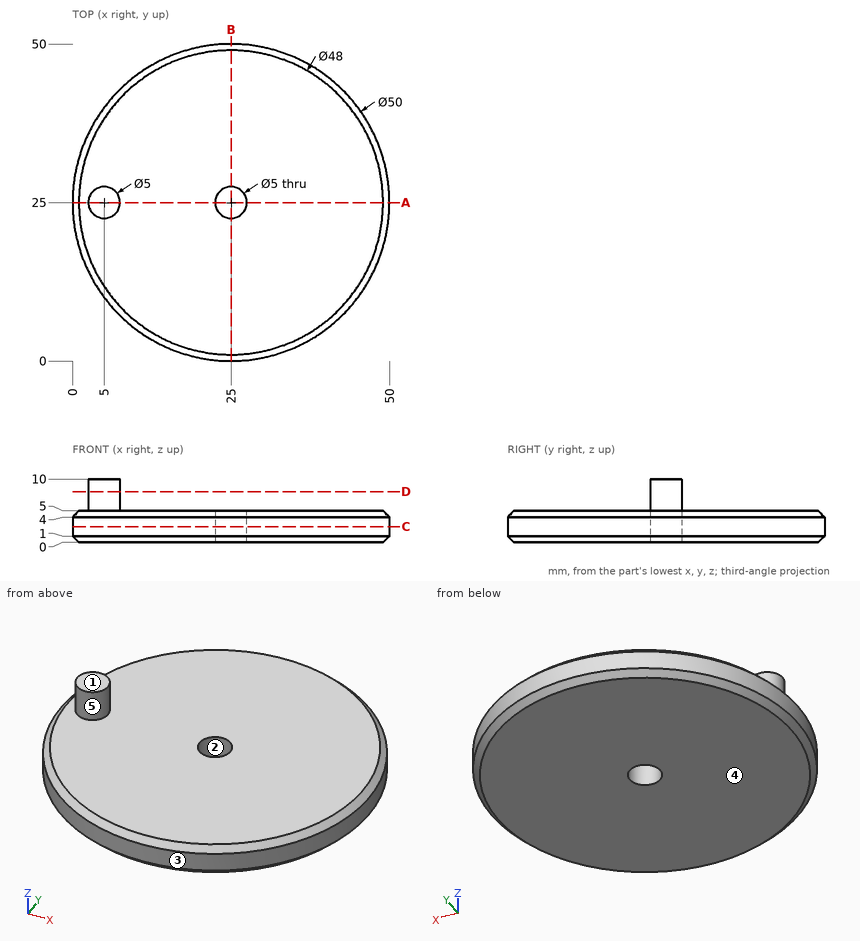
Here's the drawing with two shaded views (mm, measured from the low corner). I have some questions. A direction names the side the tool comes from. Give positions to 0.01 mm unless a question says otherwise; leave off trailing zeros. Loops run counter-clockwise (first coordinate to the right, second up) from the corner with the lowest first, then second, coordinate; pieces in that order, holes last. Notation, with made-up numbers: (63.25, 62) - (77.25, 62) arc R15 cw to (77.25, 78) - close; hole circle Ø11 at (84, 30.25). An arc over 180 degrees is marked (long way). One line per item, written item: value.
(1) If we section it at D-D, the plane z = 8: List the corners of the cut face in (x, y) for me, plus the area to 3 significant figures.
Verdict:
outline: circle Ø5 at (5, 25)
area: 19.6 mm^2
(2) If we mould it in two halves opening along Y, with no side actions, what happens to the marked faces 1, 2 and 3? For each: released by +Y, released by -Y, zero draft, split by the parting line, or undercut.
Verdict:
face 1: zero draft
face 2: undercut
face 3: split by the parting line
(3) I'm going to push flat-ended pins straight in: pin 1 (6 mm diameter, centred on x = 37.5, z = 5.5, fed in from -Y); pin 2 (2 mm diameter, centred on y = 27, z = 8, fed in from +X); pin 3 (3 mm diameter, centred on y = 34.5, z = 3.5, fed in from -X). Where does each tip first touch, or does it pass through?
Verdict:
pin 1: y = 2.04
pin 2: x = 7.29
pin 3: x = 1.31
(4) On a 3-axis mill with a long thin cutter (end or side, diameter ignored), from which of +Z, -Z, +X, -X, +Y, -Y can I reach the whole of each face in a straight line? I mean the marked faces 4 and 5. Say none if no direction works.
Verdict:
face 4: -Z, +X, -X, +Y, -Y
face 5: +Z
(5) If we section it at A-A, the plane y = 25: List the corners of the cut face in (x, z) for me.
Verdict:
outline: (0, 1) - (1, 0) - (22.5, 0) - (22.5, 5) - (7.5, 5) - (7.5, 10) - (2.5, 10) - (2.5, 5) - (1, 5) - (0, 4) - close; (27.5, 0) - (49, 0) - (50, 1) - (50, 4) - (49, 5) - (27.5, 5) - close
(6) I need wall thicknesses on line 1 along Y through (x, z) = (25, 1.35); line 2 along Z through (x, y) = (17, 14); line 3 along Y through (x, z) = (24, 2.5). Which ranges of each line are inside material? Lowest first, please.
Verdict:
line 1: 0 to 22.5, 27.5 to 50
line 2: 0 to 5
line 3: 0.02 to 22.71, 27.29 to 49.98
(7) If we section it at C-C, the plane z = 2.5: List the corners of the cut face in (x, y) for me.
Verdict:
outline: circle Ø50 at (25, 25); hole circle Ø5 at (25, 25)
(8) If we section it at B-B, the plane x = 25: List the corners of the cut face in (y, z) for me.
Verdict:
outline: (0, 1) - (1, 0) - (22.5, 0) - (22.5, 5) - (1, 5) - (0, 4) - close; (27.5, 0) - (49, 0) - (50, 1) - (50, 4) - (49, 5) - (27.5, 5) - close
